Drawing for the job (mm, zero at the part's lowest x, y, z). A direction names the side the tool comes from. Give positions to 0.01 mm unless a question says otherwise; leave off trailing zeros. Write each loop counter-clockwise with the first axis right and the second up, starting at its lowest first coordinate (ties: lowest second). Pieces come first, ordered by that corner, then holes.
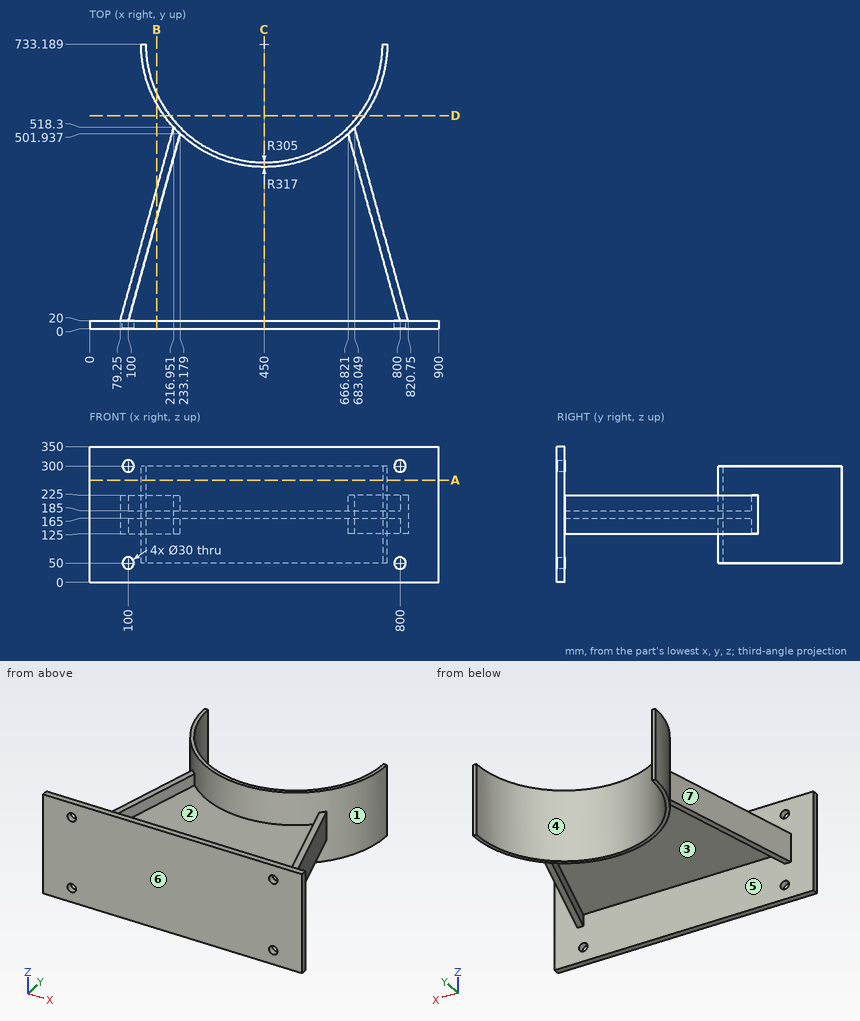
1. Slice it at A-A, the plane z = 264. Write the cut outline in (x, y).
Calculated:
outline: (0, 0) - (900, 0) - (900, 20) - (0, 20) - close; (133, 733.19) arc R317 ccw to (767, 733.19) - (755, 733.19) arc R305 cw to (145, 733.19) - close
2. Which spindle directions (+Z, -Z, +X, -X, +Y, -Y) get a long thin tool onto all of the face, cutting with end or side? Do the marked faces 1, 2, 3 and 4. Say none if no direction does.
Calculated:
face 1: none
face 2: +Z
face 3: -Z
face 4: +Z, -Z, +Y
3. Slice it at B-B, the plane x = 173. Write the cut outline in (y, z), and give its area (3 significant figures).
Calculated:
outline: (0, 0) - (20, 0) - (20, 165) - (284.17, 165) - (284.17, 125) - (359.25, 125) - (359.25, 225) - (284.17, 225) - (284.17, 185) - (20, 185) - (20, 350) - (0, 350) - close; (579.05, 50) - (605.53, 50) - (605.53, 300) - (579.05, 300) - close
area: 26,400 mm2
4. Slice it at C-C, the plane x = 450. Write the cut outline in (y, z).
Calculated:
outline: (0, 0) - (20, 0) - (20, 165) - (416.19, 165) - (416.19, 50) - (428.19, 50) - (428.19, 300) - (416.19, 300) - (416.19, 185) - (20, 185) - (20, 350) - (0, 350) - close
5. Pin check, flat tips, straight feed: P1, Ø12, axis at y = 561, z = 288, coming from the -X side (1 decimal); P2, Ø1.5, axis at x = 273, y = 218, coming from the -Z side; P3, Ø6, axis at y = 249.5, z = 163, coming from the -X side; P4, Ø18, axis at x = 800, z = 50, coming from the +Y side. Stop position of each tip, or through.
Calculated:
P1: stops at x = 180.1
P2: stops at z = 165
P3: stops at x = 141.84
P4: passes through
6. Slice it at D-D, the plane y = 549. Write the cut outline in (x, z), and give its area (3 significant figures).
Calculated:
outline: (192, 50) - (206.9, 50) - (206.9, 300) - (192, 300) - close; (693.1, 50) - (708, 50) - (708, 300) - (693.1, 300) - close
area: 7,450 mm2
7. Pull direction X, two halves, no side cores. Call the marked faces 5, 6 and 7: +X half, -X half, draft (parallel to the pull), parting line (faces both ways), or undercut.
Calculated:
face 5: undercut
face 6: draft
face 7: -X half
8. Probe probe 1 along Z at (x, y) = (800, 10.75); probe 2 along X at (y, z) = (13, 50); probe 3 along Z at (x, y) = (704, 422.5). List the from-to ranges inside material, lowest first.
Calculated:
probe 1: z = 0 to 35, 65 to 285, 315 to 350
probe 2: x = 0 to 85, 115 to 785, 815 to 900
probe 3: z = 125 to 225
